```python
from build123d import *

# Parameters (mm, degrees)
BOSS_EXTRUDE1_DEPTH = 6.35
SKETCH2_W           = 6.35
SKETCH2_H           = 25.4
CUT_EXTRUDE1_DEPTH  = 338.387086593


with BuildPart() as part:
    # Sketch1 → Boss-Extrude1 (new body)
    with BuildSketch(Plane(origin=(0, 0, 0), x_dir=(1, 0, 0), z_dir=(0, 1, 0))):
        Polygon((-42.798869448, -43.002859963), (-19.938869448, -43.002859963), (-19.938869448, -36.652859963), (5.461130552, -36.652859963), (5.461130552, -43.002859963), (28.321130552, -43.002859963), (28.321130552, -36.652859963), (53.721130552, -36.652859963), (53.721130552, -43.002859963), (76.581130552, -43.002859963), (76.581130552, -36.652859963), (101.981130552, -36.652859963), (101.981130552, -43.002859963), (124.841130552, -43.002859963), (124.841130552, -36.652859963), (150.241130552, -36.652859963), (150.241130552, -43.002859963), (173.101130552, -43.002859963), (173.101130552, -36.652859963), (198.501130552, -36.652859963), (198.501130552, -43.002859963), (212.725130552, -43.002859963), (212.725130552, 261.797140037), (198.501130552, 261.797140037), (198.501130552, 255.447140037), (173.101130552, 255.447140037), (173.101130552, 261.797140037), (150.241130552, 261.797140037), (150.241130552, 255.447140037), (124.841130552, 255.447140037), (124.841130552, 261.797140037), (101.981130552, 261.797140037), (101.981130552, 255.447140037), (76.581130552, 255.447140037), (76.581130552, 261.797140037), (53.721130552, 261.797140037), (53.721130552, 255.447140037), (28.321130552, 255.447140037), (28.321130552, 261.797140037), (5.461130552, 261.797140037), (5.461130552, 255.447140037), (-19.938869448, 255.447140037), (-19.938869448, 261.797140037), (-42.798869448, 261.797140037), (-42.798869448, 255.447140037), (-68.198869448, 255.447140037), (-68.198869448, -36.652859963), (-42.798869448, -36.652859963), align=None)
    extrude(amount=BOSS_EXTRUDE1_DEPTH)

    # Sketch2 → Cut-Extrude1 (cut, through all)
    with BuildSketch(Plane(origin=(0, 6.35, 0), x_dir=(1, 0, 0), z_dir=(0, 1, 0))):
        with Locations((44.196130552, 210.997140037)):
            Rectangle(SKETCH2_W, SKETCH2_H)
        with Locations((44.196130552, 7.797140037)):
            Rectangle(SKETCH2_W, SKETCH2_H)
        with Locations((44.196130552, 109.397140037)):
            Rectangle(SKETCH2_W, SKETCH2_H)
    extrude(amount=-CUT_EXTRUDE1_DEPTH, mode=Mode.SUBTRACT)


solid = part.part
```
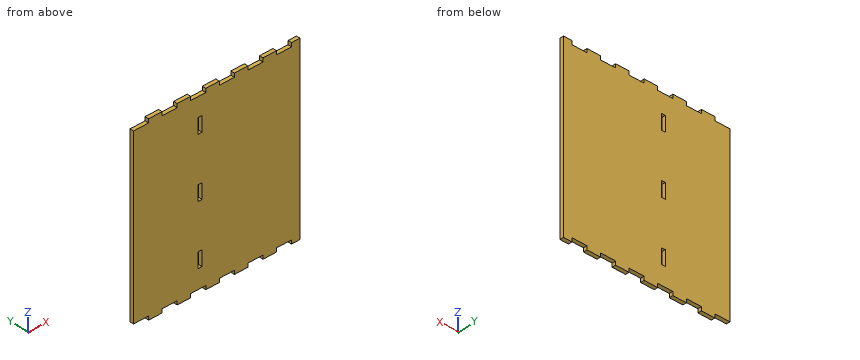
Verification items for the finished model (mm, model axes). Round coordinates to 2 decimals unless told otherwise and drop trailing zeros. Order: outer loops, then holes, each group sorted by start corner. A loop starts at its lowest first (then second) coordinate and runs counter-clockwise, first axis right, second up. Notation, with made-up numbers: (85.5, 89) -> (131.5, 89) arc R11 cw to (131.5, 98) -> close; hole circle Ø4 at (28, -20.75). An arc over 180 degrees is marked (long way). Put each result on its own line as item: value. Start each with the question number.
(1) Section check B-B (y = 5). State how many separate pieces and enclosed holes the cut face has, then the cut area to 3 significant figures.
(2) Section check A-A (z = -105.5). Enter the section's corners in (x, y), then the cut area to 3 significant figures.
(3) Section check C-C (x = 91.5). Enter the section's corners in (y, z), then the cut area to 3 significant figures.
(4) Material ranges on line 1 along X through (y, z) = (5.5, -107); line 2 along Z through (x, y) = (43.5, 3.75); line 3 along Z through (x, y) = (92.5, 4.25), recorded low to high.
(5) Depth check by flat-ended pin: pin 1 Ø3 at (x, y) = (-9, 3) entering from -Z; pin 2 Ø1.9 at (y, z) = (3.5, -259.5) entering from -X. Enter the tip coordinate at first touch or a pass-through.
Completed:
1. separate pieces: 1
1. enclosed holes: 3
1. area: 83,200 mm2
2. outline: (-68.2, 0) -> (41.02, 0) -> (41.02, 6.35) -> (-68.2, 6.35) -> close; (47.37, 0) -> (212.73, 0) -> (212.73, 6.35) -> (47.37, 6.35) -> close
2. area: 1,740 mm2
3. outline: (0, -255.45) -> (6.35, -255.45) -> (6.35, 36.65) -> (0, 36.65) -> close
3. area: 1,850 mm2
4. line 1: x = -68.2 to 41.02, 47.37 to 212.73
4. line 2: z = -255.45 to -223.7, -198.3 to -122.1, -96.7 to -20.5, 4.9 to 36.65
4. line 3: z = -255.45 to 36.65
5. pin 1: stops at z = -255.45
5. pin 2: stops at x = -42.8
